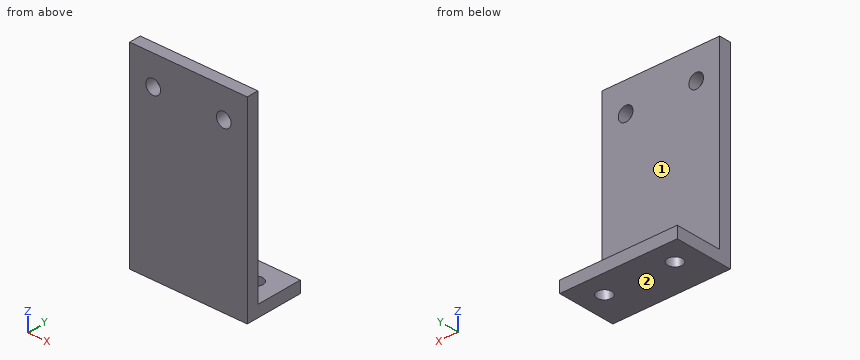
Autodesk Inventor part; units mm, degrees
ref_plane "YZ Plane" through (0, 0, 0) normal (1, 0, 0) x (0, 1, 0)
ref_plane "XZ Plane" through (0, 0, 0) normal (0, 1, 0) x (-1, 0, 0)
ref_plane "XY Plane" through (0, 0, 0) normal (0, 0, 1) x (1, 0, 0)
sketch "スケッチ1" plane through (0, 0, 0) normal (0, 0, 1) x (1, 0, 0)
  line L0 (0, 0) -> (20, 0)
  line L1 (20, 0) -> (20, 10)
  line L2 (20, 10) -> (0, 10)
  line L3 (0, 10) -> (0, 0)
  dimension "d0" = 10
  dimension "d1" = 20
extrude "押し出し1" add sketch "スケッチ1" along normal blind 2
sketch "スケッチ2" plane through (0, 0, 2) normal (0, 0, 1) x (1, 0, 0)
  line L0 (0, 10) -> (0, 0)
  line L1 (20, 0) -> (20, 10)
  line L2 (0, 0) -> (20, 0)
  line L3 (20, 0) -> (20, 2)
  line L4 (20, 2) -> (0, 2)
  line L5 (0, 2) -> (0, 0)
  point P0 (0, 2)
  dimension "d4" = 2
extrude "押し出し2" add sketch "スケッチ2" along normal blind 31.5
sketch "スケッチ3" plane through (0, 0, 2) normal (0, 0, 1) x (1, 0, 0)
  line L0 (20, 2) -> (0, 2)
  line L1 (0, 0) -> (20, 0)
  line L2 (0, 10) -> (0, 2)
  point P0 (16, 6)
  point P1 (4, 6)
  dimension "d8" = 6
  dimension "d9" = 6
  dimension "d10" = 4
  dimension "d11" = 12
hole "穴1" at (16, 6, 2) at (4, 6, 2) direction (0, 0, -1) diameter 2.5 depth 25 tip angle 118
sketch "スケッチ4" plane through (0, 2, 2) normal (0, 1, 0) x (1, 0, 0)
  line L0 (20, -31.5) -> (0, -31.5)
  line L1 (0, 0) -> (0, -31.5)
  point P0 (0, 2)
  point P1 (4, -26.5)
  point P2 (16, -26.5)
  dimension "d19" = 5
  dimension "d20" = 5
  dimension "d21" = 12
  dimension "d22" = 4
hole "穴2" at (4, 2, 28.5) at (16, 2, 28.5) direction (0, -1, 0) diameter 2.5 depth 25 tip angle 118
properties part number "シリンダ固定"
Build history of the part. All positions in model axes, mm. Face numbers are marked on the shaded views. A direction names the side the tool comes from. Coordinates: 2 decimals unless noted, no trailing zeros. Order: outer loops, then holes, each group sorted by start corner. A loop starts at its lowest first (then second) coordinate and runs counter-clockwise, first axis right, second up. Notation, with made-up numbers: (-33, -37) - (-6, -37) arc R22 cw to (-6, -5) - close; hole circle Ø8 at (36.5, 42.25). An arc over 180 degrees is marked (long way). Put each result on its own line as item: value.
1. Tool access for the marked faces 1 and 2: list every direction of +Z, -Z, +X, -X, +Y, -Y with a clear straight run to the whole face (end or side of a thin tool).
Answer sheet:
face 1: +Z, +X, -X, +Y
face 2: -Z, +X, -X, +Y, -Y
2. Saw through at A-A (y = 6). Write the cut outline in (x, z), and give its area (3 significant figures).
Answer sheet:
outline: (0, 0) - (2.75, 0) - (2.75, 2) - (0, 2) - close; (5.25, 0) - (14.75, 0) - (14.75, 2) - (5.25, 2) - close; (17.25, 0) - (20, 0) - (20, 2) - (17.25, 2) - close
area: 30.0 mm^2
3. Probe line 1 along X through (y, z) = (6, 0.8); line 2 along Y through (x, z) = (16, 1.55); line 3 along Z through (x, y) = (4, 0.55). List the from-to ranges inside material, lowest first. Write a range as [from, to].
Answer sheet:
line 1: x = [0, 2.75], [5.25, 14.75], [17.25, 20]
line 2: y = [0, 4.75], [7.25, 10]
line 3: z = [0, 27.25], [29.75, 33.5]
4. Drop flat-ended pins along their axis: P1, Ø4, axis at x = 8, y = 6, coming from the +Z side; P2, Ø2, axis at x = 16, z = 28.5, coming from the -Y side; P3, Ø10, axis at x = 14, z = 24.5, coming from the +Y side. Give the stop position or say it passes through.
Answer sheet:
P1: stops at z = 2
P2: passes through
P3: stops at y = 2
5. Saw through at C-C (x = 4). Write the cut outline in (y, z).
Answer sheet:
outline: (0, 0) - (4.75, 0) - (4.75, 2) - (2, 2) - (2, 27.25) - (0, 27.25) - close; (0, 29.75) - (2, 29.75) - (2, 33.5) - (0, 33.5) - close; (7.25, 0) - (10, 0) - (10, 2) - (7.25, 2) - close
6. Saw through at D-D (y = 2.75). Write the cut outline in (x, z).
Answer sheet:
outline: (0, 0) - (20, 0) - (20, 2) - (0, 2) - close
